from build123d import *
from build123d.topology import SkipClean

# Parameters (mm, degrees)
SKETCH1_R           = 30.05
SKETCH1_R_2         = 28.55
BOSS_EXTRUDE1_DEPTH = 3
BOSS_EXTRUDE2_START = -3
SKETCH1_3_R         = 30.05
SKETCH1_3_R_2       = 28.55
BOSS_EXTRUDE2_DEPTH = 3
BOSS_EXTRUDE3_START = 25
BOSS_EXTRUDE3_DEPTH = 25
SKETCH4_W           = 0.7
SKETCH4_H           = 5
CUT_EXTRUDE1_START  = -0.5
CUT_EXTRUDE1_DEPTH  = 0.5


# Read off the part's stored shape, not the designer's step: Cut-Extrude1
with BuildPart() as part:
    # Sketch1 → Boss-Extrude1 (new body)
    # profile 1 of 2: a face of its own
    with BuildSketch(Plane.XY):
        Circle(SKETCH1_R)
        Circle(SKETCH1_R_2, mode=Mode.SUBTRACT)
    # profile 2 of 2: a face of its own
    with BuildSketch(Plane.XY):
        Circle(SKETCH1_R_2)
    extrude(amount=BOSS_EXTRUDE1_DEPTH)

    # Sketch1<3> → Boss-Extrude2 (add)
    with BuildSketch(Plane.XY.offset(BOSS_EXTRUDE2_START)):
        Circle(SKETCH1_3_R)
        Circle(SKETCH1_3_R_2, mode=Mode.SUBTRACT)
    extrude(amount=BOSS_EXTRUDE2_DEPTH)

    # Sketch3 → Boss-Extrude3 (add)
    with SkipClean():  # the faces are left unmerged after this step: merging them gives an invalid solid
        with BuildSketch(Plane(origin=(0, 0, -3), x_dir=(-1, 0, 0), z_dir=(0, 0, -1)).offset(BOSS_EXTRUDE3_START)):
            with BuildLine():
                Line((20.491380882, 21.979668094), (19.468516612, 20.882513281))
                ThreePointArc((19.468516612, 20.882513281), (10.461996603, 26.564057052), (0, 28.55))
                Line((0, 28.55), (0, 30.05))
                ThreePointArc((0, 30.05), (11.011663675, 27.959716793), (20.491380882, 21.979668094))
            make_face()
            with BuildLine():
                Line((30.031566735, 1.05237798), (28.532486865, 0.999846633))
                ThreePointArc((28.532486865, 0.999846633), (26.18137362, 11.385876135), (20.187898603, 20.187898603))
                Line((20.187898603, 20.187898603), (21.248558775, 21.248558775))
                ThreePointArc((21.248558775, 21.248558775), (27.5569274, 11.984083288), (30.031566735, 1.05237798))
            make_face()
            with BuildLine():
                Line((21.979668094, -20.491380882), (20.882513281, -19.468516612))
                ThreePointArc((20.882513281, -19.468516612), (26.564057052, -10.461996603), (28.55, 0))
                Line((28.55, 0), (30.05, 0))
                ThreePointArc((30.05, 0), (27.959716793, -11.011663675), (21.979668094, -20.491380882))
            make_face()
            with BuildLine():
                Line((1.05237798, -30.031566735), (0.999846633, -28.532486865))
                ThreePointArc((0.999846633, -28.532486865), (11.385876135, -26.18137362), (20.187898603, -20.187898603))
                Line((20.187898603, -20.187898603), (21.248558775, -21.248558775))
                ThreePointArc((21.248558775, -21.248558775), (11.984083288, -27.5569274), (1.05237798, -30.031566735))
            make_face()
            with BuildLine():
                Line((-20.491380882, -21.979668094), (-19.468516612, -20.882513281))
                ThreePointArc((-19.468516612, -20.882513281), (-10.461996603, -26.564057052), (0, -28.55))
                Line((0, -28.55), (0, -30.05))
                ThreePointArc((0, -30.05), (-11.011663675, -27.959716793), (-20.491380882, -21.979668094))
            make_face()
            with BuildLine():
                Line((-30.031566735, -1.05237798), (-28.532486865, -0.999846633))
                ThreePointArc((-28.532486865, -0.999846633), (-26.18137362, -11.385876135), (-20.187898603, -20.187898603))
                Line((-20.187898603, -20.187898603), (-21.248558775, -21.248558775))
                ThreePointArc((-21.248558775, -21.248558775), (-27.5569274, -11.984083288), (-30.031566735, -1.05237798))
            make_face()
            with BuildLine():
                Line((-21.979668094, 20.491380882), (-20.882513281, 19.468516612))
                ThreePointArc((-20.882513281, 19.468516612), (-26.564057052, 10.461996603), (-28.55, 0))
                Line((-28.55, 0), (-30.05, 0))
                ThreePointArc((-30.05, 0), (-27.959716793, 11.011663675), (-21.979668094, 20.491380882))
            make_face()
            with BuildLine():
                Line((-1.05237798, 30.031566735), (-0.999846633, 28.532486865))
                ThreePointArc((-0.999846633, 28.532486865), (-11.385876135, 26.18137362), (-20.187898603, 20.187898603))
                Line((-20.187898603, 20.187898603), (-21.248558775, 21.248558775))
                ThreePointArc((-21.248558775, 21.248558775), (-11.984083288, 27.5569274), (-1.05237798, 30.031566735))
            make_face()
        extrude(amount=-BOSS_EXTRUDE3_DEPTH)

    # Sketch4 → Cut-Revolve1 (revolve, cut)
    with SkipClean():  # the faces are left unmerged after this step: merging them gives an invalid solid
        with BuildSketch(Plane(origin=(0, 0, 0), x_dir=(1, 0, 0), z_dir=(0, 1, 0))):
            with Locations((29.7, 22.5)):
                Rectangle(SKETCH4_W, SKETCH4_H)
            Polygon((28.55, 26.5), (28.55, 28), (30.05, 28), align=None)
        revolve(axis=Axis((0, 0, 3), (0, 0, -1)), mode=Mode.SUBTRACT)

    # Cut-Extrude1 outline → Cut-Extrude1 (cut)
    # profile 1 of 4: a face of its own
    with SkipClean():  # the faces are left unmerged after this step: merging them gives an invalid solid
        with BuildSketch(Plane.XY.offset(3).offset(CUT_EXTRUDE1_START)):
            with BuildLine():
                add(Edge.make_bspline(
                    [(-9.831188481, -7.76286267), (-12.31509908, -6.564453694), (-19.945506052, -1.751090116), (-23.245520708, 3.604062551), (-24.465440518, 11.416266415), (-15.133909058, 13.3540246), (-0.220085461, 12.125105625), (7.518774259, 6.992670667), (9.641745648, 5.518604803)],
                    knots=[0, 0, 0, 0, 0.123562004, 0.211727559, 0.248485922, 0.454387264, 0.532112439, 1, 1, 1, 1], degree=3))
                add(Edge.make_bspline(
                    [(-9.831188481, -7.76286267), (-14.608290319, -3.536611009), (-17.897696817, -0.898578419), (-21.378258226, 5.519092244), (-19.304554183, 8.268748828)],
                    knots=[0, 0, 0, 0, 0.497115956, 0.99999998, 0.99999998, 0.99999998, 0.99999998], degree=3))
                add(Edge.make_bspline(
                    [(9.641745648, 5.518604803), (-12.302292658, 17.553494797), (-19.304554183, 8.268748828)],
                    knots=[1.224732712, 1.224732712, 1.224732712, 3.011762383, 3.011762383, 3.011762383], degree=2, weights=[1, 0.626676865, 1]))
            make_face()
        # profile 2 of 4: a face of its own
        with BuildSketch(Plane.XY.offset(3).offset(CUT_EXTRUDE1_START)):
            with BuildLine():
                add(Edge.make_bspline(
                    [(9.831188481, 7.76286267), (12.31509908, 6.564453694), (19.945506052, 1.751090116), (23.245520708, -3.604062551), (24.465440518, -11.416266415), (15.133909058, -13.3540246), (0.220085461, -12.125105625), (-7.518774259, -6.992670667), (-9.641745648, -5.518604803)],
                    knots=[0, 0, 0, 0, 0.123562004, 0.211727559, 0.248485922, 0.454387264, 0.532112439, 1, 1, 1, 1], degree=3))
                add(Edge.make_bspline(
                    [(9.831188481, 7.76286267), (14.608290319, 3.536611009), (17.897696883, 0.898578367), (21.378258365, -5.5190925), (19.304553936, -8.268749156)],
                    knots=[0, 0, 0, 0, 0.497115956, 1, 1, 1, 1], degree=3))
                add(Edge.make_bspline(
                    [(-9.641745648, -5.518604803), (12.302291673, -17.553494257), (19.304553936, -8.268749156)],
                    knots=[4.366325366, 4.366325366, 4.366325366, 6.153354993, 6.153354993, 6.153354993], degree=2, weights=[1, 0.626676882, 1]))
            make_face()
        # profile 3 of 4: a face of its own
        with BuildSketch(Plane.XY.offset(3).offset(CUT_EXTRUDE1_START)):
            with BuildLine():
                add(Edge.make_bspline(
                    [(-16.054779318, 5.843461789), (-19.839576992, -4.555184358), (6.134990822, -8.121053968), (32.109558636, -11.686923579), (9.919788496, 2.277592179), (-12.269981644, 16.242107937), (-16.054779318, 5.843461789)],
                    knots=[0, 0, 0, 2.094395102, 2.094395102, 4.188790205, 4.188790205, 6.283185307, 6.283185307, 6.283185307], degree=2, weights=[1, 0.5, 1, 0.5, 1, 0.5, 1]))
            make_face()
            with BuildLine():
                add(Edge.make_bspline(
                    [(-11.355964711, 4.133233136), (-13.640122053, -2.142437584), (4.535903685, -5.204451928), (22.711929422, -8.266466273), (6.820061027, 1.071218792), (-9.071807369, 10.408903856), (-11.355964711, 4.133233136)],
                    knots=[0, 0, 0, 2.094395102, 2.094395102, 4.188790205, 4.188790205, 6.283185307, 6.283185307, 6.283185307], degree=2, weights=[1, 0.5, 1, 0.5, 1, 0.5, 1]))
            make_face(mode=Mode.SUBTRACT)
        # profile 4 of 4: a face of its own
        with BuildSketch(Plane.XY.offset(3).offset(CUT_EXTRUDE1_START)):
            with BuildLine():
                add(Edge.make_bspline(
                    [(-0.545917498, -1.499895999), (1.967945144, -2.431945071), (5.077041498, -3.030895568), (6.737953902, -1.750447632), (1.605929106, 4.537470773), (-6.123195001, 3.076782229), (-6.04339485, 1.101123427), (-3.081000207, -0.559979297), (-0.545917498, -1.499895999)],
                    knots=[0, 0, 0, 0, 0.245515964, 0.295417536, 0.499015724, 0.702313155, 0.752411582, 1, 1, 1, 1], degree=3))
            make_face()
        extrude(amount=CUT_EXTRUDE1_DEPTH, mode=Mode.SUBTRACT)


solid = part.part
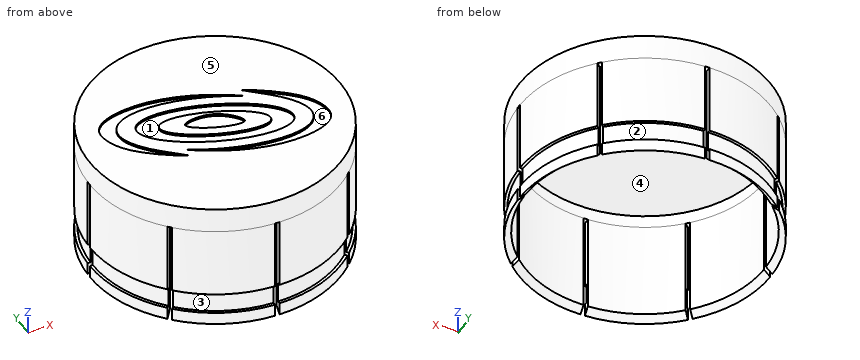
Here's how the part is built. I have some questions about the finished solid (model axes, mm). Face numbers are marked on the shaded views. A direction names the side the tool comes from. Coordinates: 2 decimals unless noted, no trailing zeros.
1) I'm going to push flat-ended pins straight in: pin 1 (3 mm diameter, centred on x = -20, y = -7, fed in from -Z); pin 2 (6 mm diameter, centred on x = -11.5, z = -9, fed in from -Y); pin 3 (0.5 mm diameter, centred on x = 21.5, y = 20.5, fed in from -Z). Where does each tip first touch, or does it pass through?
Filled in:
pin 1: stops at z = 0
pin 2: stops at y = -28.82
pin 3: stops at z = -3
2) Thinking about a two-plate mould opening in X: for the marked faces 1, 2 and 3, which applies, +X half, -X half, draft (parallel to the pull), parting line (faces both ways), or undercut?
Filled in:
face 1: undercut
face 2: +X half
face 3: -X half
3) If we section it at A-A (z = -11): Count the separate pieces of the cut face and the enclosed holes in it, plus the area to 3 significant figures.
Filled in:
separate pieces: 8
enclosed holes: 0
area: 264 mm2
4) If I drill on line 1 (Y direction, x = 0, z = -1.2); line 2 (X direction, y = -21, z = -8.5); line 3 (X direction, y = -9.5, z = -22.5), over which ranges is the centre line in solid material (lowest first)?
Filled in:
line 1: y = -30.05 to -28.55, 28.55 to 30.05
line 2: x = -21 to -19.34, 19.34 to 19.58, 21 to 21.49
line 3: x = -27.77 to -26.92, 26.92 to 27.77
5) Which directions (+Z, -Z, +X, -X, +Y, -Y) give clear straight access to the entire face, cutting with the end or side of a thin tool? Please do the marked faces 4, 5 and 6.
Filled in:
face 4: -Z
face 5: +Z, +X, -X, +Y, -Y
face 6: +Z
